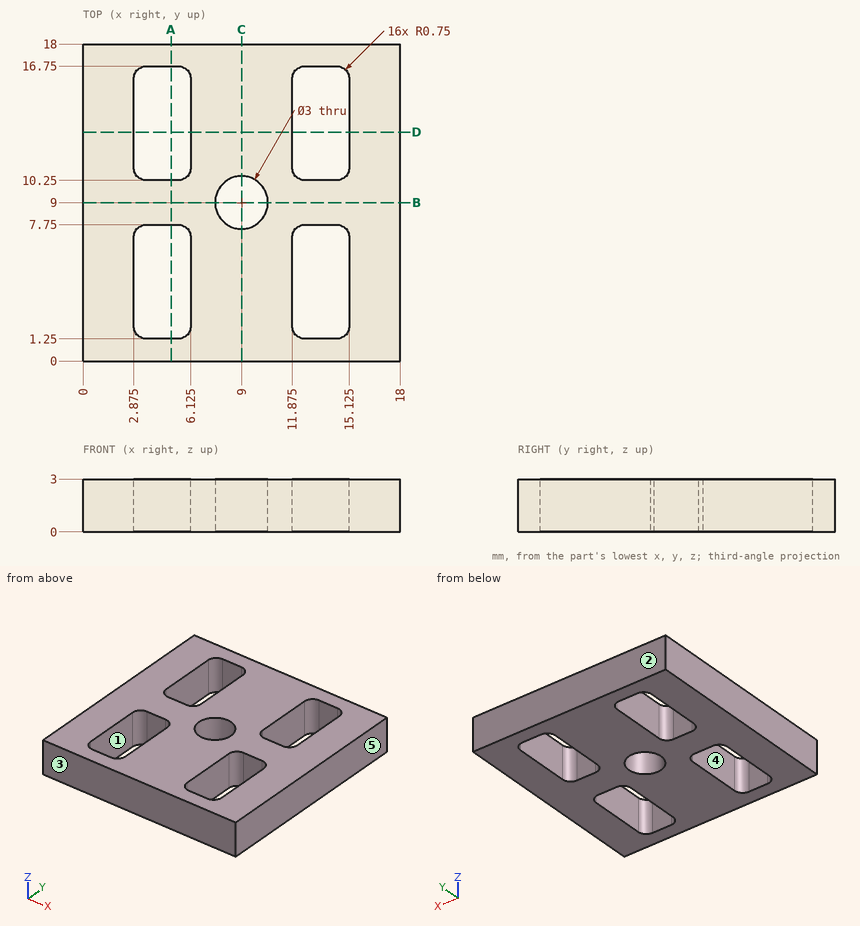
Here's the drawing with two shaded views (mm, measured from the low corner). I have some questions. A direction names the side the tool comes from. Coordinates: 2 decimals unless noted, no trailing zeros. Write each loop counter-clockwise with the first axis right and the second up, starting at its lowest first coordinate (ties: lowest second). Pieces come first, ordered by that corner, then holes. Notation, with made-up numbers: M -20.5,-4.75 L 15.5,-4.75 A20 cw 15.5,26.25 Z; hole C 36,26.5 d10. An arc over 180 degrees is marked long. Answer as CSV lines item,"result". Start each with the question number.
1) We'd pull the mould along Y, two halves only. Please class the marked faces 1, 2 and 3: +Y half, -Y half, draft (parallel to the pull), parting line (faces both ways), or undercut.
2) I want a section at B-B, the plane y = 9. Please give me the cut outline in (x, z).
3) I want a section at A-A, the plane x = 5. Please give me the cut outline in (y, z), and give its area (3 significant figures).
4) For the marked faces 4 and 5, which set-ups out of +Z, -Z, +X, -X, +Y, -Y let a thin tool reach every point of the face, with its end or its side?
5) Please list where these lines run through material, in increasing order: line 1 (X direction, y = 16, z = 2.3) (3 decimals); line 2 (Y direction, x = 4, z = 2); line 3 (Y direction, x = 9, z = 2.05). Write a range as from..to.
6) I want a section at D-D, the plane y = 13. Please give me the cut outline in (x, z) (3 decimals).
Data:
1,face 1,"undercut"
1,face 2,"+Y half"
1,face 3,"-Y half"
2,outline,"M 0,0 L 7.5,0 L 7.5,3 L 0,3 Z; M 10.5,0 L 18,0 L 18,3 L 10.5,3 Z"
3,outline,"M 0,0 L 1.25,0 L 1.25,3 L 0,3 Z; M 7.75,0 L 10.25,0 L 10.25,3 L 7.75,3 Z; M 16.75,0 L 18,0 L 18,3 L 16.75,3 Z"
3,area,"15.0 mm^2"
4,face 4,"+Z, -Z"
4,face 5,"+Z, -Z, +X, +Y, -Y"
5,line 1,"x = 0..2.875, 6.125..11.875, 15.125..18"
5,line 2,"y = 0..1.25, 7.75..10.25, 16.75..18"
5,line 3,"y = 0..7.5, 10.5..18"
6,outline,"M 0,0 L 2.875,0 L 2.875,3 L 0,3 Z; M 6.125,0 L 11.875,0 L 11.875,3 L 6.125,3 Z; M 15.125,0 L 18,0 L 18,3 L 15.125,3 Z"
